```python
from build123d import *

# Parameters (mm, degrees)
SZKIC1_R                    = 5
DODANIE_WYCI_GNI_CIE1_DEPTH = 3


with BuildPart() as part:
    # Szkic1 → Dodanie-wyciągnięcie1 (new body)
    with BuildSketch(Plane(origin=(0, 0, -1.5), x_dir=(-1, 0, 0), z_dir=(0, 0, -1))):
        with BuildLine():
            Line((-12, 0), (-12, -23.217670017))
            Line((-12, -23.217670017), (-10.5, -23.217670017))
            ThreePointArc((-10.5, -23.217670017), (0, -17.5), (10.5, -23.217670017))
            Line((10.5, -23.217670017), (12, -23.217670017))
            Line((12, -23.217670017), (12, 0))
            ThreePointArc((12, 0), (0, 12), (-12, 0))
        make_face()
        Circle(SZKIC1_R, mode=Mode.SUBTRACT)
    extrude(amount=-DODANIE_WYCI_GNI_CIE1_DEPTH)


solid = part.part
```
Input: part model. Units: mm. Frame: model coordinates. Coordinates: 2 decimals unless noted, no trailing zeros. Write each loop counter-clockwise with the first axis right and the second up, starting at its lowest first coordinate (ties: lowest second). Pieces come first, ordered by that corner, then holes.
1) Section D-D on y = 7. Output: boundary loops of the cut face in (x, z).
2) Section A-A on z = -0.85. Output: boundary loops of the cut face in (x, y).
3) Material intervals for line 1 along Y through (x, z) = (0, -0.8); line 2 along Y through (x, z) = (-3.75, -1.2); line 3 along X through (y, z) = (-18.5, -1), sorted ascending.
4) Section B-B on y = -3.5. Output: boundary loops of the cut face in (x, z), and give its area (3 significant figures).
5) Mould query, pull axis X, two halves, no side actions, for faces 1 (the flat face through (-12, -12, 0)), 2 (the cylindrical face through (1.08, -4.88, -0.02)), 3 (the flat face through (-11, -23.218, 0)). Classes: pulls with the +X half, pulls with the -X half, needs draft (parallel to the pull), parting line crosses it, or undercut.
6) Section C-C on x = 3.75. Output: boundary loops of the cut face in (y, z).
Check result:
1. outline: (-9.75, -1.5) - (9.75, -1.5) - (9.75, 1.5) - (-9.75, 1.5) - close
2. outline: (-12, -23.22) - (-10.5, -23.22) arc R12.5 cw to (10.5, -23.22) - (12, -23.22) - (12, 0) arc R12 ccw to (-12, 0) - close; hole circle Ø10 at (0, 0)
3. line 1: y = -17.5 to -5, 5 to 12
3. line 2: y = -18.08 to -3.31, 3.31 to 11.4
3. line 3: x = -12 to -4.9, 4.9 to 12
4. outline: (-12, -1.5) - (-3.57, -1.5) - (-3.57, 1.5) - (-12, 1.5) - close; (3.57, -1.5) - (12, -1.5) - (12, 1.5) - (3.57, 1.5) - close
4. area: 50.6 mm2
5. face 1: pulls with the -X half
5. face 2: undercut
5. face 3: needs draft
6. outline: (-18.08, -1.5) - (-3.31, -1.5) - (-3.31, 1.5) - (-18.08, 1.5) - close; (3.31, -1.5) - (11.4, -1.5) - (11.4, 1.5) - (3.31, 1.5) - close
